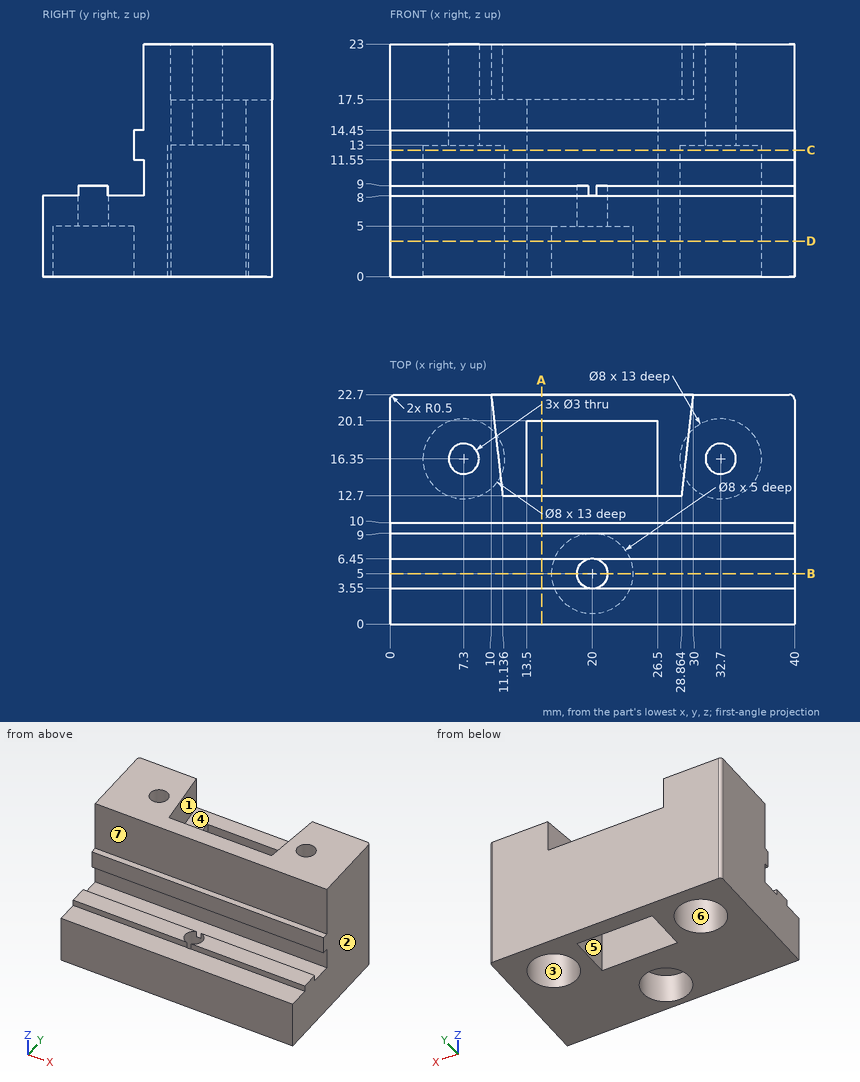
Here's the drawing with two shaded views (mm, measured from the low corner). I have some questions. A direction names the side the tool comes from. Round coordinates to 2 decimals unless told otherwise and drop trailing zeros. Write each loop counter-clockwise with the first axis right and the second up, starting at its lowest first coordinate (ties: lowest second). Pieces come first, ordered by that corner, then holes. Notation, with made-up numbers: M 31,-16 L 66,-16 A23 ccw 66,-4 Z; hole C -37.75,81 d6. An arc over 180 degrees is marked long. Write each question's results on one line, items separated by ' | '. Start each with the question number.
1. Imagine slicing it at C-C on z = 12.5. List the corners of the cut face in (x, y) for me, and give its area (3 significant figures).
2. Imagine slicing it at D-D on z = 3.5. List the corners of the cut face in (x, y) for me.
3. Thinking about a two-plate mould opening in Y: for the marked faces 1, 2 and 3, which applies, +Y half, -Y half, draft (parallel to the pull), parting line (faces both ways), or undercut?
4. On a 3-axis mill with a long thin cutter (end or side, diameter ignored), from which of +Z, -Z, +X, -X, +Y, -Y can I reach the whole of each face in a straight line? I mean the marked faces 4, 5, 6 and 7. Say none if no direction works.
5. I need wall thicknesses on L1, parallel to Y at x = 20, z = 7.95; L2, parallel to X at y = 15.75, z = 7.75 (1 decimal); L3, parallel to Y at x = 20, z = 8.25. Which ranges of each line are inside material? Lowest first, please. Write a range as from..to.
6. Imagine slicing it at A-A on x = 15. List the corners of the cut face in (y, z) for me, and give its area (3 significant figures).
7. Imagine slicing it at B-B on y = 5. List the corners of the cut face in (x, z) for me.
8. I'm going to push flat-ended pins straight in: pin 1 Ø1.8 at (x, z) = (24, 10) entering from -Y; pin 2 Ø0.9 at (x, y) = (6.5, 5) entering from +Z; pin 3 Ø0.9 at (x, z) = (13, 13) entering from -Y. Where does each tip first touch, or does it pass through?
Result sheet:
1) outline: M 0,9 L 40,9 L 40,22.2 A0.5 ccw 39.5,22.7 L 0.5,22.7 A0.5 ccw 0,22.2 Z; hole C 7.3,16.35 d8; hole M 13.5,12.7 L 26.5,12.7 L 26.5,20.1 L 13.5,20.1 Z; hole C 32.7,16.35 d8 | area: 351 mm^2
2) outline: M 0,0 L 40,0 L 40,22.2 A0.5 ccw 39.5,22.7 L 0.5,22.7 A0.5 ccw 0,22.2 Z; hole C 7.3,16.35 d8; hole M 13.5,12.7 L 26.5,12.7 L 26.5,20.1 L 13.5,20.1 Z; hole C 20,5 d8; hole C 32.7,16.35 d8
3) face 1: +Y half | face 2: draft | face 3: undercut
4) face 4: +Z, +Y | face 5: +Z, -Z | face 6: -Z | face 7: +Z, +X, -X, -Y
5) L1: y = 0..3.5, 6.5..12.7, 20.1..22.7 | L2: x = 0..3.3, 11.3..13.5, 26.5..28.7, 36.7..40 | L3: y = 10..12.7, 20.1..22.7
6) outline: M 0,0 L 12.7,0 L 12.7,23 L 10,23 L 10,14.45 L 9,14.45 L 9,11.55 L 10,11.55 L 10,8 L 6.45,8 L 6.45,9 L 3.55,9 L 3.55,8 L 0,8 Z; M 20.1,0 L 22.7,0 L 22.7,17.5 L 20.1,17.5 Z | area: 193 mm^2
7) outline: M 0,0 L 16,0 L 16,5 L 18.5,5 L 18.5,9 L 0,9 Z; M 21.5,5 L 24,5 L 24,0 L 40,0 L 40,9 L 21.5,9 Z
8) pin 1: stops at y = 10 | pin 2: stops at z = 9 | pin 3: stops at y = 9
